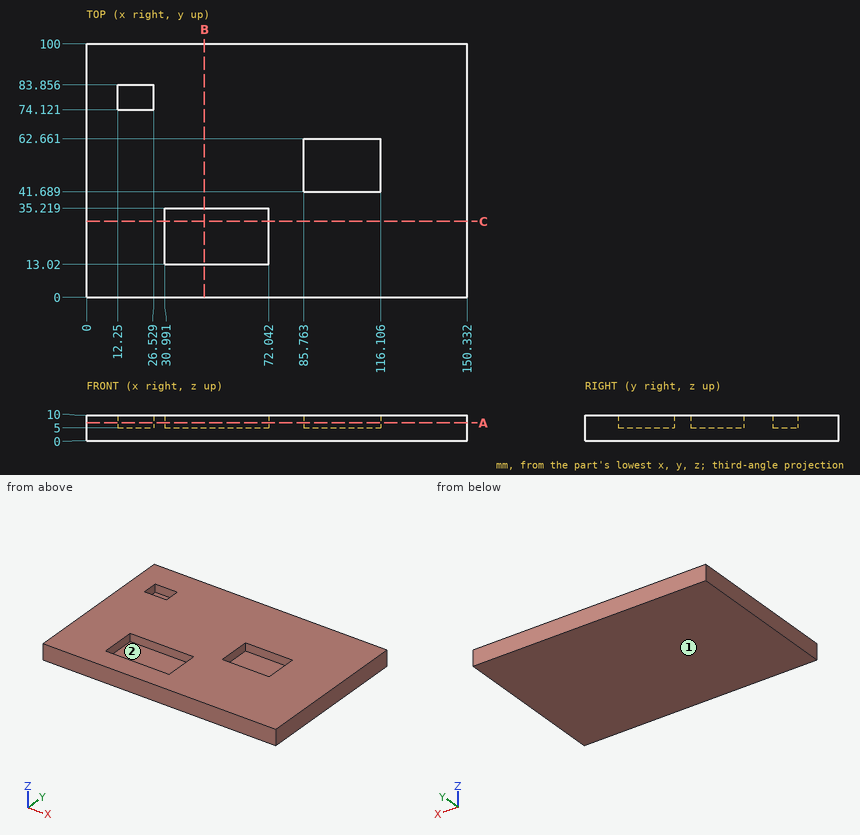
Geometry: see drawing. Coordinates: mm, zero at the bounding-box minimum. Round coordinates to 2 decimals unless told otherwise and drop trailing zeros. Loops run counter-clockwise (first coordinate to the right, second up) from the corner with the lowest first, then second, coordinate; pieces in that order, holes last. Notation, with made-up numbers: M -30.75,9.5 L 4.25,9.5 A19 cw 4.25,44.5 Z; hole C 52.25,69 d10. An arc over 180 degrees is marked long. Use a Markdown table: item, result. Add a question column.
1. Cut plane A-A, the plane z = 7. State how many separate pieces and enclosed holes the cut face has, and give its area (3 significant figures).
2. Contact query for a flat-ended pin moving along its axis: pin 1 (10.5 mm diameter, centred on x = 99, y = 55.5, fed in from +Z). Output: stop coordinate, or through.
3. Ray query, line 1 along Y through (x, z) = (111.5, 8.5); line 2 along X through (y, z) = (57.5, 5.5) (1 decimal); line 3 along X through (y, z) = (81, 7.75). Return the intervals inside material, ascending. Write a range as [from, to].
4. Cut plane B-B, the plane x = 46.5. Output: boundary loops of the cut face in (y, z).
5. Pull-direction query (Y, two-part tool) for the marked faces 1 and 2; classes: +Y half, -Y half, draft (parallel to the pull), parting line (faces both ways), or undercut.
6. Cut plane C-C, the plane y = 30. Output: boundary loops of the cut face in (x, z).
Solution:
| question | item | result |
|---|---|---|
| 1 | separate pieces | 1 |
| 1 | enclosed holes | 3 |
| 1 | area | 13,300 mm2 |
| 2 | pin 1 | stops at z = 5 |
| 3 | line 1 | y = [0, 41.69], [62.66, 100] |
| 3 | line 2 | x = [0, 85.8], [116.1, 150.3] |
| 3 | line 3 | x = [0, 12.25], [26.53, 150.33] |
| 4 | outline | M 0,0 L 100,0 L 100,10 L 35.22,10 L 35.22,5 L 13.02,5 L 13.02,10 L 0,10 Z |
| 5 | face 1 | draft |
| 5 | face 2 | undercut |
| 6 | outline | M 0,0 L 150.33,0 L 150.33,10 L 72.04,10 L 72.04,5 L 30.99,5 L 30.99,10 L 0,10 Z |
